Part model, mm, in its own coordinate system. A direction names the side the tool comes from. Give positions to 0.01 mm unless a question says otherwise; leave off trailing zeros. Write each loop counter-clockwise with the first axis right and the second up, starting at its lowest first coordinate (ties: lowest second). Pieces come first, ordered by that corner, then holes. Notation, with made-up numbers: M -17,-39.75 L 14,-39.75 A18 cw 14,-12.75 Z; hole C 40.5,68 d6. An arc over 180 degrees is marked long. Use CSV: the item, a comma, the result in double quotes. Start each with the question number.
Item 1: Cut at B-B (y = 15.5). List the corners of the cut face in (x, z) (3 decimals).
Item 2: Cut at C-C (z = 0). List the corners of the cut face in (x, y) (3 decimals).
Item 3: Pin check, flat tips, straight feed: pin 1 (10 mm diameter, centred on y = 13.5, z = 6, fed in from +X); pin 2 (4.5 mm diameter, centred on y = 16, z = -5.5, fed in from +X); pin 3 (3 mm diameter, centred on y = 7, z = 5.5, fed in from +X); pin 4 (0.5 mm diameter, centred on x = -14.5, y = 11.5, fed in from -Z). Stop position of each tip, or through.
Item 4: Drill centre lines: line 1 (Z direction, x = -2, y = 16.75) (3 decimals); line 2 (Z direction, x = 0.5, y = 1); line 3 (Z direction, x = 3.5, y = 11.5). Where is each one in solid material? Low to high. Write a range as [from, to].
Item 5: Cut at D-D (y = 6.25). List the corners of the cut face in (x, z).
Item 6: Cut at A-A (x = -9.5). List the corners of the cut face in (y, z) (3 decimals), then the cut area to 3 significant figures.
Item 7: Which spindle directions (+Z, -Z, +X, -X, +Y, -Y) get a long thin tool onto all of the face, cutting with end or side? Do faces 4 (the flat face through (-14.3, 9, 0)), 5 (the flat face through (14.3, 9, 0)), 6 (the flat face through (-7, 9, 15.3)), 7 (the flat face through (-7, 9, -15.3)), 8 (the flat face through (-6, 15, -12.925)). Say none if no direction does.
Item 8: Mould opens along Z. For faces 1 (the cylindrical face through (0.383, 16.424, 14.076)), 2 (the cylindrical face through (-14.7, 9.37, 14.73)), 3 (the cylindrical face through (-12.355, 14.563, -12.324)) say: released by +Z, released by -Z, zero draft, split by the parting line, or undercut.
from build123d import *

# Parameters (mm, degrees)
BOSS_EXTRUDE1_DEPTH     = 19
CUT_EXTRUDE1_DEPTH      = 9
CUT_EXTRUDE2_DEPTH      = 29.795485757
CUT_EXTRUDE2_DEPTH_BACK = 29.795485757
SKETCH3_R               = 1
SKETCH8_W               = 1
SKETCH8_H               = 3
CUT_EXTRUDE9_DEPTH      = 29.79548593


with BuildPart() as part:
    # Sketch1 → Boss-Extrude1 (new body)
    with BuildSketch(Plane(origin=(0, 0, 0), x_dir=(1, 0, 0), z_dir=(0, 1, 0))):
        with BuildLine():
            Line((-13.3, 15.3), (0, 15.3))
            ThreePointArc((0, 15.3), (15.3, 0), (0, -15.3))
            Line((0, -15.3), (-13.3, -15.3))
            ThreePointArc((-13.3, -15.3), (-14.714213562, -14.714213562), (-15.3, -13.3))
            Line((-15.3, -13.3), (-15.3, 13.3))
            ThreePointArc((-15.3, 13.3), (-14.714213562, 14.714213562), (-13.3, 15.3))
        make_face()
    extrude(amount=BOSS_EXTRUDE1_DEPTH)

    # Sketch2 → Cut-Extrude1 (cut)
    with BuildSketch(Plane(origin=(0, 19, 0), x_dir=(1, 0, 0), z_dir=(0, 1, 0))):
        with BuildLine():
            Line((-10.925, 12.925), (0, 12.925))
            ThreePointArc((0, 12.925), (12.925, 0), (0, -12.925))
            Line((0, -12.925), (-10.925, -12.925))
            ThreePointArc((-10.925, -12.925), (-12.339213562, -12.339213562), (-12.925, -10.925))
            Line((-12.925, -10.925), (-12.925, 10.925))
            ThreePointArc((-12.925, 10.925), (-12.339213562, 12.339213562), (-10.925, 12.925))
        make_face()
    extrude(amount=-CUT_EXTRUDE1_DEPTH, mode=Mode.SUBTRACT)

    # Sketch3 → Cut-Extrude2 (cut, two sides: drawn at the far end of the back side and taken through both)
    with BuildSketch(Plane.XY.offset(-CUT_EXTRUDE2_DEPTH_BACK)):
        with Locations(Location((0, 15.5, 0), (0, 0, 90))):
            Circle(SKETCH3_R)
    extrude(amount=CUT_EXTRUDE2_DEPTH + CUT_EXTRUDE2_DEPTH_BACK, mode=Mode.SUBTRACT)

    # Sketch8 → Cut-Extrude9 (cut, through all)
    with BuildSketch(Plane(origin=(0, 0, 0), x_dir=(1, 0, 0), z_dir=(0, 1, 0))):
        with Locations((14.8, 0)):
            Rectangle(SKETCH8_W, SKETCH8_H)
        with Locations((-14.8, 0)):
            Rectangle(SKETCH8_W, SKETCH8_H)
    extrude(amount=CUT_EXTRUDE9_DEPTH, mode=Mode.SUBTRACT)


solid = part.part
Worked answers:
1,outline,"M -15.3,-13.3 A2 ccw -13.3,-15.3 L -1,-15.3 L -1,-12.925 L -10.925,-12.925 A2 cw -12.925,-10.925 L -12.925,10.925 A2 cw -10.925,12.925 L -1,12.925 L -1,15.3 L -13.3,15.3 A2 ccw -15.3,13.3 L -15.3,1.5 L -14.3,1.5 L -14.3,-1.5 L -15.3,-1.5 Z; M 1,-15.267 A15.3 ccw 15.226,-1.5 L 14.3,-1.5 L 14.3,1.5 L 15.226,1.5 A15.3 ccw 1,15.267 L 1,12.886 A12.925 cw 1,-12.886 Z"
2,outline,"M -14.3,0 L 14.3,0 L 14.3,19 L 12.925,19 L 12.925,10 L -12.925,10 L -12.925,19 L -14.3,19 Z"
3,pin 1,"stops at x = 15.23"
3,pin 2,"stops at x = 14.95"
3,pin 3,"stops at x = 14.77"
3,pin 4,"stops at z = -15.06"
4,line 1,"z = [-15.3, -12.925], [12.925, 15.3]"
4,line 2,"z = [-15.29, 15.29]"
4,line 3,"z = [-14.89, -12.44], [12.44, 14.89]"
5,outline,"M -15.3,-13.3 A2 ccw -13.3,-15.3 L 0,-15.3 A15.3 ccw 15.23,-1.5 L 14.3,-1.5 L 14.3,1.5 L 15.23,1.5 A15.3 ccw 0,15.3 L -13.3,15.3 A2 ccw -15.3,13.3 L -15.3,1.5 L -14.3,1.5 L -14.3,-1.5 L -15.3,-1.5 Z"
6,outline,"M 0,-15.3 L 19,-15.3 L 19,-12.925 L 10,-12.925 L 10,12.925 L 19,12.925 L 19,15.3 L 0,15.3 Z"
6,area,"349 mm^2"
7,face 4,"-X, +Y, -Y"
7,face 5,"+X, +Y, -Y"
7,face 6,"+Z, +X, -X, +Y, -Y"
7,face 7,"-Z, +X, -X, +Y, -Y"
7,face 8,"+Y"
8,face 1,"zero draft"
8,face 2,"released by +Z"
8,face 3,"undercut"
